Read the model definition and answer for the solid it produces. Units are mm, in the model's axes. A direction names the side the tool comes from. Round coordinates to 2 decimals unless told otherwise and drop trailing zeros. Order: outer loops, then holes, each group sorted by start corner. A loop starts at its lowest first (then second) coordinate and runs counter-clockwise, first axis right, second up. Notation, with made-up numbers: (28.5, 88) -> (74.5, 88) arc R36 ccw to (74.5, 127) -> close; hole circle Ø9 at (-1.5, 89). An arc over 180 degrees is marked (long way). Answer as a JSON object with one key per item and string values. Group by question number.
Item 1: Consider probe 1 along Z at (x, y) = (22, -2063.5); probe 2 along X at (y, z) = (-539.5, 84); probe 3 along Y at (x, z) = (-36.5, 104.5). Determine where each line is inside the solid, lowest interval first. Write a range as from..to.
Item 2: Section B-B, the plane y = -1124 is taken. Write down the section's boundary in (x, z).
Item 3: For faces 1 (the flat face through (11.483, -1428, 27)), 2 (the flat face through (-3, -1428, 127.593)), 3 (the flat face through (-18.517, -1428, 28)), determine the directions among +Z, -Z, +X, -X, +Y, -Y from which every point of the face is accessible in a straight line to the end or side of a thin tool.
Item 4: Section A-A, the plane z = -6.5 is taken. Write down the section's boundary in (x, y), plus the area to 3 significant figures.
Item 5: Given P1, Ø4, axis at y = -2433, z = 63.5, coming from the +X side; P2, Ø1, axis at y = -1447, z = -26.5, coming from the -X side, each flat-ended and moving along its own axis, determine where each tip first touches the part or whether it passes through.
from build123d import *

# Parameters (mm, degrees)
F1_DEPTH = 2900
F2_R     = 8
F3_R     = 5


with BuildPart() as f1:
    # F0 (on Front) → F1 (new body)
    with BuildSketch(Plane.XZ):
        Polygon((36.482626, 127.592679), (-43.517374, 127.592679), (-43.517374, 87.592679), (-18.517374, 87.592679), (-18.517374, -32.407321), (-43.517374, -32.407321), (-43.517374, -72.407321), (36.482626, -72.407321), (36.482626, -32.407321), (11.482626, -32.407321), (11.482626, 87.592679), (36.482626, 87.592679), align=None)
    extrude(amount=F1_DEPTH)

    # F2
    f2_edges = [f1.edges().sort_by_distance(p)[0] for p in [
        (-3.517374, -2900, 127.592679),
        (-43.517374, -2900, 107.592679),
        (-31.017374, -2900, 87.592679),
        (-18.517374, -2900, 27.592679),
        (-31.017374, -2900, -32.407321),
        (-43.517374, -2900, -52.407321),
        (-3.517374, -2900, -72.407321),
        (36.482626, -2900, -52.407321),
        (23.982626, -2900, -32.407321),
        (11.482626, -2900, 27.592679),
        (23.982626, -2900, 87.592679),
        (36.482626, -2900, 107.592679),
    ]]
    fillet(f2_edges, radius=F2_R)

    # F3
    f3_edges = [f1.edges().sort_by_distance(p)[0] for p in [
        (-3.517374, 0, 127.592679),
        (-43.517374, 0, 107.592679),
        (-31.017374, 0, 87.592679),
        (-18.517374, 0, 27.592679),
        (-31.017374, 0, -32.407321),
        (-43.517374, 0, -52.407321),
        (-3.517374, 0, -72.407321),
        (36.482626, 0, -52.407321),
        (23.982626, 0, -32.407321),
        (11.482626, 0, 27.592679),
        (23.982626, 0, 87.592679),
        (36.482626, 0, 107.592679),
    ]]
    fillet(f3_edges, radius=F3_R)


solid = f1.part
Values found:
{
 "1": {"probe 1": "-72.41..-32.41, 87.59..127.59", "probe 2": "-18.52..11.48", "probe 3": "-2899.94..0"},
 "2": {"outline": "(-43.52, -72.41) -> (36.48, -72.41) -> (36.48, -32.41) -> (11.48, -32.41) -> (11.48, 87.59) -> (36.48, 87.59) -> (36.48, 127.59) -> (-43.52, 127.59) -> (-43.52, 87.59) -> (-18.52, 87.59) -> (-18.52, -32.41) -> (-43.52, -32.41) -> close"},
 "3": {"face 1": "+X, +Y, -Y", "face 2": "+Z, +X, -X, +Y, -Y", "face 3": "-X, +Y, -Y"},
 "4": {"outline": "(-18.52, -2892) arc R8 ccw to (-10.52, -2900) -> (3.48, -2900) arc R8 ccw to (11.48, -2892) -> (11.48, -5) arc R5 ccw to (6.48, 0) -> (-13.52, 0) arc R5 ccw to (-18.52, -5) -> close", "area": "87,000 mm2"},
 "5": {"P1": "x = 11.48", "P2": "x = -18.52"}
}
